```python
from build123d import *

# Parameters (mm, degrees)
F0_W      = 60.96
F0_H      = 104.14
F0_R      = 17.78
F0_R_2    = 7.62
F1_DEPTH  = 6.35
F2_R      = 17.7657824196
F2_R_2    = 7.588336925
F3_DEPTH  = 0.254
F4_W      = 52.7304011778
F4_H      = 38.1
F5_DEPTH  = 0.254
F6_W      = 7.5248517096
F6_H      = 2.2023727652
F7_DEPTH  = 0.762
F8_R      = 5.08
F9_R      = 0.6248874124
F10_DEPTH = 0.1
F11_W     = 17.3393432051
F11_H     = 0.9681868833
F12_DEPTH = 0.1
F13_R     = 0.2460151655
F13_R_2   = 0.2460152488
F13_R_3   = 0.2218778153
F13_R_4   = 0.2339087287
F13_R_5   = 0.2167167574
F14_DEPTH = 0.2


with BuildPart() as f1:
    # F0 (on Front) → F1 (new body)
    with BuildSketch(Plane.XZ):
        with Locations((-0.6015785038, 6.9682898942)):
            Rectangle(F0_W, F0_H)
        with Locations((0, -14.6217101058)):
            Circle(F0_R, mode=Mode.SUBTRACT)
        Polygon((-26.619868353, 33.6382898942), (-26.619868353, 52.6882898942), (25.7174987346, 52.6882898942), (25.7174987346, 14.5882898942), (-26.619868353, 14.5882898942), align=None, mode=Mode.SUBTRACT)
        Polygon((25.7174987346, 52.6882898942), (-26.619868353, 52.6882898942), (-26.619868353, 33.6382898942), (-26.619868353, 14.5882898942), (25.7174987346, 14.5882898942), align=None)
        with Locations((0, -14.6217101058)):
            Circle(F0_R)
        with Locations((0, -14.6217101058)):
            Circle(F0_R_2, mode=Mode.SUBTRACT)
        with Locations((0, -14.6217101058)):
            Circle(F0_R_2)
    extrude(amount=F1_DEPTH)

    # F2 (on face) → F3 (join)
    with BuildSketch(Plane.XZ.offset(6.35)):
        with Locations((0, -14.6216154099)):
            Circle(F2_R)
        with Locations((0, -14.6216154099)):
            Circle(F2_R_2, mode=Mode.SUBTRACT)
    extrude(amount=F3_DEPTH)

    # F4 (on face) → F5 (join)
    with BuildSketch(Plane.XZ.offset(6.35)):
        with Locations((-0.6015794352, 33.9892106131)):
            Rectangle(F4_W, F4_H)
    extrude(amount=F5_DEPTH)

    # F6 (on face) → F7 (join)
    with BuildSketch(Plane.XY.offset(59.0382898942)):
        with Locations((-21.2724506855, -4.1166004958)):
            Rectangle(F6_W, F6_H)
    extrude(amount=F7_DEPTH)

    # F8
    f8_edges = [f1.edges().sort_by_distance(p)[0] for p in [
        (29.878421, -3.175, 59.03829),
        (-31.081579, -3.175, 59.03829),
        (-31.081579, -3.175, -45.10171),
        (29.878421, -3.175, -45.10171),
    ]]
    fillet(f8_edges, radius=F8_R)

    # F9 (on face) → F10 (cut)
    with BuildSketch(Plane.XY.offset(59.0382898942)):
        with Locations((21.9533834606, -3.6403015256)):
            Circle(F9_R)
    extrude(amount=-F10_DEPTH, mode=Mode.SUBTRACT)

    # F11 (on face) → F12 (cut)
    with BuildSketch(Plane(origin=(0, 0, -45.1017101058), x_dir=(1, 0, 0), z_dir=(0, 0, -1))):
        with Locations((0.1725424081, 3.2033285825)):
            Rectangle(F11_W, F11_H)
    extrude(amount=-F12_DEPTH, mode=Mode.SUBTRACT)

    # F13 (on face) → F14 (cut)
    with BuildSketch(Plane(origin=(0, 0, -45.0017101058), x_dir=(1, 0, 0), z_dir=(0, 0, -1))):
        with Locations((-6.265850272, 3.1648736913)):
            Circle(F13_R)
        with Locations((-3.4933153074, 3.1428695656)):
            Circle(F13_R_2)
        with Locations((0, 3.1428695656)):
            Circle(F13_R_3)
        with Locations((3.5260387231, 3.1428695656)):
            Circle(F13_R_4)
        with Locations((7.1127302945, 3.1428695656)):
            Circle(F13_R_5)
    extrude(amount=-F14_DEPTH, mode=Mode.SUBTRACT)


solid = f1.part
```
Here's how the part is built. I have some questions about the finished solid (model axes, mm). A direction names the side the tool comes from. Coordinates: 2 decimals unless noted, no trailing zeros. Write each loop counter-clockwise with the first axis right and the second up, starting at its lowest first coordinate (ties: lowest second). Pieces come first, ordered by that corner, then holes. Notation, with made-up numbers: M 15.25,-5.75 L 64.25,-5.75 A18 ccw 64.25,1.25 Z; hole C 1.5,7 d2. An arc over 180 degrees is marked long. Answer as CSV lines item,"result". Start each with the question number.
Q1. Suppose I cut it at B-B, the plane z = 4.5. List the corners of the cut face in (x, y) for me.
Q2. Suppose I cut it at A-A, the plane x = -20. List the corners of the cut face in (y, z) for me, then the cut area to 3 significant figures.
Q3. If we mould it in two halves opening along Z, with no side actions, what happens to faces 3 (the flat face through (-1, -4, -45.102)), 4 (the flat face through (-1, -6.604, 34)), 5 (the flat face through (-21, -4, 59.8)), 6 (the flat face through (-1, -6.35, 8))? For each: pulls with the +Z half, pulls with the -Z half, needs draft (parallel to the pull), parting line crosses it, or undercut.
Q4. For faces 1 (the cylindrical face through (-29.633, -3.219, 57.511)), 2 (the flat face through (0, -6.35, -15)), which set-ups out of +Z, -Z, +X, -X, +Y, -Y let a thin tool reach every point of the face, with its end or its side?
Q5. Will these pins go through, and if not, where does the flat tip stop? pin 1 Ø0.8 at (y, z) = (-4, 59.5) entering from +X; pin 2 Ø3 at (x, y) = (-8, -3.5) entering from +Z; pin 3 Ø0.8 at (y, z) = (-4, 59.5) entering from -X.
Q6. Suppose I cut it at C-C, the plane x = 12. List the corners of the cut face in (y, z) for me.
Q7. I need wall thicknesses on probe 1 along Z at (x, y) = (0, -6.5); probe 2 along Z at (x, y) = (-9, -2); probe 3 along Y at (x, z) = (-15, 10). Which ranges of each line are inside material? Lowest first, please. Write a range as [from, to].
Entries:
1,outline,"M -31.08,-6.35 L 29.88,-6.35 L 29.88,0 L -31.08,0 Z"
2,outline,"M -6.6,14.94 L -6.35,14.94 L -6.35,-45.1 L 0,-45.1 L 0,59.04 L -3.02,59.04 L -3.02,59.8 L -5.22,59.8 L -5.22,59.04 L -6.35,59.04 L -6.35,53.04 L -6.6,53.04 Z"
2,area,"673 mm²"
3,face 3,"pulls with the -Z half"
3,face 4,"needs draft"
3,face 5,"pulls with the +Z half"
3,face 6,"undercut"
4,face 1,"+Z, -X, +Y, -Y"
4,face 2,"-Y"
5,pin 1,"stops at x = -17.51"
5,pin 2,"stops at z = 59.04"
5,pin 3,"stops at x = -25.03"
6,outline,"M -6.6,-27.72 L -6.35,-27.72 L -6.35,-45.1 L 0,-45.1 L 0,59.04 L -6.35,59.04 L -6.35,53.04 L -6.6,53.04 L -6.6,14.94 L -6.35,14.94 L -6.35,-1.52 L -6.6,-1.52 Z"
7,probe 1,"z = [-32.39, -22.21], [-7.03, 3.14], [14.94, 53.04]"
7,probe 2,"z = [-45.1, 59.04]"
7,probe 3,"y = [-6.35, 0]"
